For this review, take the finished solid that the model builds, in its own axes (mm). Face numbers are marked on the shaded views. A direction names the side the tool comes from. Give positions to 0.01 mm unless a question says otherwise; leave off trailing zeros. Order: outer loops, then holes, each group sorted by start corner. A loop starts at its lowest first (then second) coordinate and runs counter-clockwise, first axis right, second up. Notation, with made-up numbers: (-6.5, 22) - (-1.5, 22) arc R15 cw to (-1.5, 40) - close; hole circle Ø8 at (-38, 49). An arc over 180 degrees is marked (long way). One line per item, written item: value.
```python
from build123d import *

# Parameters (mm, degrees)
SKETCH_W        = 60
SKETCH_H        = 30
PAD_DEPTH       = 20
SKETCH001_W     = 14
SKETCH001_H     = 5
POCKET_DEPTH    = 20.001
SKETCH002_W     = 14
SKETCH002_H     = 5
POCKET001_DEPTH = 20.001
SKETCH003_W     = 38
SKETCH003_H     = 20
POCKET002_DEPTH = 20.001
SKETCH005_W     = 38
SKETCH005_H     = 5
POCKET003_DEPTH = 20.001
SKETCH006_W     = 9
SKETCH006_H     = 3
POCKET004_DEPTH = 20.001
SKETCH007_W     = 1
SKETCH007_H     = 4
POCKET005_DEPTH = 20.001
SKETCH008_W     = 30
SKETCH008_H     = 18
POCKET006_DEPTH = 5
FILLET_R        = 1
FILLET001_R     = 1
FILLET002_R     = 1
FILLET003_R     = 1
FILLET004_R     = 1
FILLET005_R     = 1
FILLET006_R     = 1
FILLET007_R     = 1
SKETCH011_W     = 20
SKETCH011_H     = 18
POCKET007_DEPTH = 10
SKETCH012_W     = 20
SKETCH012_H     = 18
POCKET008_DEPTH = 10
FILLET008_R     = 1
FILLET009_R     = 1
SKETCH014_W     = 6
SKETCH014_H     = 10
POCKET009_DEPTH = 60.001
SKETCH015_R     = 1.5
POCKET010_DEPTH = 5
SKETCH016_R     = 1.5
POCKET011_DEPTH = 60.001
PAD001_DEPTH    = 3
FILLET010_R     = 1
FILLET011_R     = 1
FILLET012_R     = 1
FILLET013_R     = 1


with BuildPart() as part:
    # Sketch → Pad (new body)
    with BuildSketch(Plane.XZ):
        with Locations((30, 15)):
            Rectangle(SKETCH_W, SKETCH_H)
    extrude(amount=PAD_DEPTH)

    # Sketch001 (on Face6 of Pad) → Pocket (cut, through all)
    with BuildSketch(Plane.XZ.offset(20)):
        with Locations((8, 3.5)):
            Rectangle(SKETCH001_W, SKETCH001_H)
    extrude(amount=-POCKET_DEPTH, mode=Mode.SUBTRACT)

    # Sketch002 (on Face5 of Pocket) → Pocket001 (cut, through all)
    with BuildSketch(Plane.XZ.offset(20)):
        with Locations((52, 3.5)):
            Rectangle(SKETCH002_W, SKETCH002_H)
    extrude(amount=-POCKET001_DEPTH, mode=Mode.SUBTRACT)

    # Sketch003 (on Face5 of Pocket001) → Pocket002 (cut, through all)
    with BuildSketch(Plane.XZ.offset(20)):
        with Locations((30, 16)):
            Rectangle(SKETCH003_W, SKETCH003_H)
    extrude(amount=-POCKET002_DEPTH, mode=Mode.SUBTRACT)

    # Sketch005 (on Face5 of Pocket002) → Pocket003 (cut, through all)
    with BuildSketch(Plane.XZ.offset(20)):
        with Locations((30, 28.5)):
            Rectangle(SKETCH005_W, SKETCH005_H)
    extrude(amount=-POCKET003_DEPTH, mode=Mode.SUBTRACT)

    # Sketch006 (on Face5 of Pocket003) → Pocket004 (cut, through all)
    with BuildSketch(Plane.XZ.offset(20)):
        with Locations((5.5, 27.5)):
            Rectangle(SKETCH006_W, SKETCH006_H)
        with Locations((54.5, 27.5)):
            Rectangle(SKETCH006_W, SKETCH006_H)
    extrude(amount=-POCKET004_DEPTH, mode=Mode.SUBTRACT)

    # Sketch007 (on Face5 of Pocket004) → Pocket005 (cut, through all)
    with BuildSketch(Plane.XZ.offset(20)):
        with Locations((10.5, 28)):
            Rectangle(SKETCH007_W, SKETCH007_H)
        with Locations((49.5, 28)):
            Rectangle(SKETCH007_W, SKETCH007_H)
    extrude(amount=-POCKET005_DEPTH, mode=Mode.SUBTRACT)

    # Sketch008 (on Face18 of Pocket005) → Pocket006 (cut)
    with BuildSketch(Plane(origin=(0, 0, 6), x_dir=(-1, 0, 0), z_dir=(0, 0, 1))):
        with Locations((-30, 10)):
            Rectangle(SKETCH008_W, SKETCH008_H)
    extrude(amount=-POCKET006_DEPTH, mode=Mode.SUBTRACT)

    # Fillet
    fillet_edges = [part.edges().sort_by_distance(p)[0] for p in [
        (60, -10, 0),
    ]]
    fillet(fillet_edges, radius=FILLET_R)

    # Fillet001
    fillet001_edges = [part.edges().sort_by_distance(p)[0] for p in [
        (0, -10, 0),
    ]]
    fillet(fillet001_edges, radius=FILLET001_R)

    # Fillet002
    fillet002_edges = [part.edges().sort_by_distance(p)[0] for p in [
        (0, -10, 30),
    ]]
    fillet(fillet002_edges, radius=FILLET002_R)

    # Fillet003
    fillet003_edges = [part.edges().sort_by_distance(p)[0] for p in [
        (60, -10, 30),
    ]]
    fillet(fillet003_edges, radius=FILLET003_R)

    # Fillet004
    fillet004_edges = [part.edges().sort_by_distance(p)[0] for p in [
        (1, -10, 29),
    ]]
    fillet(fillet004_edges, radius=FILLET004_R)

    # Fillet005
    fillet005_edges = [part.edges().sort_by_distance(p)[0] for p in [
        (1, -10, 1),
    ]]
    fillet(fillet005_edges, radius=FILLET005_R)

    # Fillet006
    fillet006_edges = [part.edges().sort_by_distance(p)[0] for p in [
        (59, -10, 29),
    ]]
    fillet(fillet006_edges, radius=FILLET006_R)

    # Fillet007
    fillet007_edges = [part.edges().sort_by_distance(p)[0] for p in [
        (59, -10, 1),
    ]]
    fillet(fillet007_edges, radius=FILLET007_R)

    # Sketch011 (on Face6 of Fillet007) → Pocket007 (cut)
    with BuildSketch(Plane(origin=(49, 0, 0), x_dir=(0, 0, -1), z_dir=(-1, 0, 0))):
        with Locations((-16, 10)):
            Rectangle(SKETCH011_W, SKETCH011_H)
    extrude(amount=-POCKET007_DEPTH, mode=Mode.SUBTRACT)

    # Sketch012 (on Face21 of Pocket007) → Pocket008 (cut)
    with BuildSketch(Plane(origin=(11, 0, 0), x_dir=(0, 0, 1), z_dir=(1, 0, 0))):
        with Locations((16, 10)):
            Rectangle(SKETCH012_W, SKETCH012_H)
    extrude(amount=-POCKET008_DEPTH, mode=Mode.SUBTRACT)

    # Fillet008
    fillet008_edges = [part.edges().sort_by_distance(p)[0] for p in [
        (30, -19, 1),
    ]]
    fillet(fillet008_edges, radius=FILLET008_R)

    # Fillet009
    fillet009_edges = [part.edges().sort_by_distance(p)[0] for p in [
        (30, -1, 1),
    ]]
    fillet(fillet009_edges, radius=FILLET009_R)

    # Sketch014 (on Face33 of Fillet009) → Pocket009 (cut, through all)
    with BuildSketch(Plane(origin=(60, 0, 0), x_dir=(0, 0, 1), z_dir=(1, 0, 0))):
        with Locations((4, 10)):
            Rectangle(SKETCH014_W, SKETCH014_H)
    extrude(amount=-POCKET009_DEPTH, mode=Mode.SUBTRACT)

    # Sketch015 (on Face32 of Pocket009) → Pocket010 (cut)
    with BuildSketch(Plane(origin=(0, 0, 0), x_dir=(1, 0, 0), z_dir=(0, 0, -1))):
        with Locations((55, 5)):
            Circle(SKETCH015_R)
        with Locations((55, 15)):
            Circle(SKETCH015_R)
        with Locations((5, 5)):
            Circle(SKETCH015_R)
        with Locations((5, 15)):
            Circle(SKETCH015_R)
    extrude(amount=-POCKET010_DEPTH, mode=Mode.SUBTRACT)

    # Sketch016 (on Face30 of Pocket010) → Pocket011 (cut, through all)
    with BuildSketch(Plane(origin=(0, 0, 0), x_dir=(0, 0, -1), z_dir=(-1, 0, 0))):
        with Locations((-15.994056, 9.992209)):
            Circle(SKETCH016_R)
    extrude(amount=-POCKET011_DEPTH, mode=Mode.SUBTRACT)

    # Sketch017 (on Face32 of Pocket011) → Pad001 (join)
    with BuildSketch(Plane(origin=(0, 0, 0), x_dir=(1, 0, 0), z_dir=(0, 0, -1))):
        Polygon((59, 20), (59, 40), (1, 40), (1, 20), (1, 0), (1, -20), (59, -20), (59, 0), align=None)
    extrude(amount=PAD001_DEPTH)

    # Fillet010
    fillet010_edges = [part.edges().sort_by_distance(p)[0] for p in [
        (59, -40, -1.5),
    ]]
    fillet(fillet010_edges, radius=FILLET010_R)

    # Fillet011
    fillet011_edges = [part.edges().sort_by_distance(p)[0] for p in [
        (1, 20, -1.5),
    ]]
    fillet(fillet011_edges, radius=FILLET011_R)

    # Fillet012
    fillet012_edges = [part.edges().sort_by_distance(p)[0] for p in [
        (59, 20, -1.5),
    ]]
    fillet(fillet012_edges, radius=FILLET012_R)

    # Fillet013
    fillet013_edges = [part.edges().sort_by_distance(p)[0] for p in [
        (1, -40, -1.5),
    ]]
    fillet(fillet013_edges, radius=FILLET013_R)


solid = part.part
```
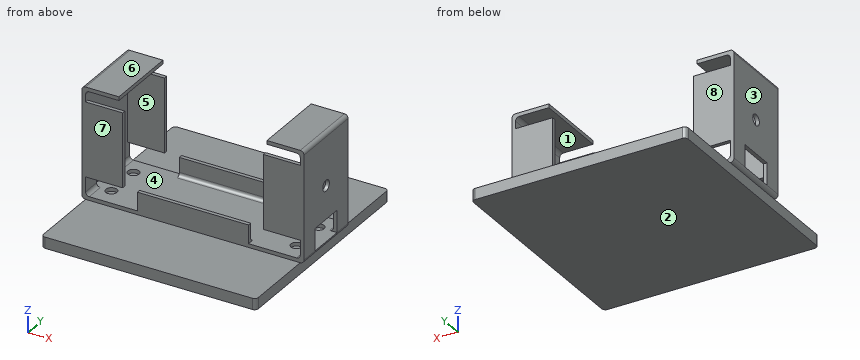
(1) Machinability: for the marked faces 5, 6, 7 and 8, which of the approach directions +Z, -Z, +X, -X, +Y, -Y give a long, thin tool a straight path to every point of the face, cutting with its end or side? Answer none if there is none.
Answers below:
face 5: none
face 6: +Z, +X, -X, +Y, -Y
face 7: +Z, +X, -X, -Y
face 8: +Z, +X, -X, +Y
(2) Draft analysis for pull direction Z (two halves, no side actions). For the marked faces 1, 2, 3 and 4, state which applies: pulls with the +Z half, pulls with the -Z half, needs draft (parallel to the pull), parting line crosses it, or undercut.
Answers below:
face 1: undercut
face 2: pulls with the -Z half
face 3: needs draft
face 4: undercut
(3) Take a section at B-B (y = -12.5). Write out the cut boundary in (x, z), then the cut area to 3 significant figures.
Answers below:
outline: (0, 1) arc R1 ccw to (1, 0) - (1, -3) - (59, -3) - (59, 0) arc R1 ccw to (60, 1) - close; (0, 7) - (1, 7) - (1, 28) arc R1 cw to (2, 29) - (10, 29) - (10, 30) - (1, 30) arc R1 ccw to (0, 29) - close; (50, 29) - (58, 29) arc R1 cw to (59, 28) - (59, 7) - (60, 7) - (60, 29) arc R1 ccw to (59, 30) - (50, 30) - close
area: 298 mm^2
(4) Take a section at D-D (x = 22). Write out the cut boundary in (y, z).
Answers below:
outline: (-40, -3) - (20, -3) - (20, 0) - (0, 0) - (0, 6) - (-1, 6) - (-1, 2) arc R1 cw to (-2, 1) - (-18, 1) arc R1 cw to (-19, 2) - (-19, 6) - (-20, 6) - (-20, 0) - (-40, 0) - close
(5) Take a section at C-C (x = 5). Write out the cut boundary in (y, z), then the cut area to 3 significant figures.
Answers below:
outline: (-40, -3) - (20, -3) - (20, 0) - (0, 0) - (0, 1) - (-3.5, 1) - (-3.5, 0) - (-6.5, 0) - (-6.5, 1) - (-13.5, 1) - (-13.5, 0) - (-16.5, 0) - (-16.5, 1) - (-20, 1) - (-20, 0) - (-40, 0) - close; (-20, 6) - (-19, 6) - (-19, 26) - (-20, 26) - close; (-20, 29) - (0, 29) - (0, 30) - (-20, 30) - close; (-1, 6) - (0, 6) - (0, 26) - (-1, 26) - close
area: 254 mm^2
(6) Wall thickness on line 1 (Y direction, x = 55, z = 0.45); line 2 (X direction, y = -7, z = 18.5); line 3 (Y direction, x = 5.5, z = 24.5): over which ranges is each line inside the solid? List them lowest first. Write a range as from..to.
Answers below:
line 1: y = -20..-16.5, -13.5..-6.5, -3.5..0
line 2: x = 0..1, 59..60
line 3: y = -20..-19, -1..0
(7) Take a section at A-A (z = 19). Write out the cut boundary in (x, y), then the cut area to 3 significant figures.
Answers below:
outline: (0, -20) - (11, -20) - (11, -19) - (1, -19) - (1, -1) - (11, -1) - (11, 0) - (0, 0) - close; (49, -20) - (60, -20) - (60, 0) - (49, 0) - (49, -1) - (59, -1) - (59, -19) - (49, -19) - close
area: 80.0 mm^2
(8) For P1, Ø1, axis at x = 59, z = 3, coming from the +Y side; P2, Ø15, axis at x = 17, z = 17, coming from the -Y side; P3, Ø1.5, axis at y = -6.5, z = -1, coming from the +X side, all flat-tipped, find the tip position at first contact; note any pin that passes through.
Answers below:
P1: stops at y = 0
P2: stops at y = -20
P3: stops at x = 59
